Geometry check sheet. Reference: the model listing, model coordinates, mm. A direction names the side the tool comes from. Coordinates: 2 decimals unless noted, no trailing zeros. Order: outer loops, then holes, each group sorted by start corner. A loop starts at its lowest first (then second) coordinate and runs counter-clockwise, first axis right, second up. Notation, with made-up numbers: M -28.75,-32.75 L -2.75,-32.75 A27 cw -2.75,2.25 Z; hole C 18,7 d5. An arc over 180 degrees is marked long. One line per item, written item: value. Start each with the question number.
1) Sectioned sample at A-A, the plane z = -6.25. Enter the section's corners in (x, y), then the cut area to 3 significant figures.
2) Sectioned sample at C-C, the plane x = 1. Enter the section's corners in (y, z), then the cut area to 3 significant figures.
3) Go/stop test with flat-tipped pins: P1, Ø2.5, axis at x = 31.91, y = -16.6, coming from the +Z side; P2, Ø1.5, axis at x = 6.5, y = -8.5, coming from the -Z side; P3, Ø6, axis at x = -33, z = 1.5, coming from the +Y side; P4, Ø2, axis at y = 9, z = 1, coming from the -X side. Record where each tip stops, or that it passes through.
4) Draft check along X on faces 1 (the cylindrical face through (-21.994, -5.777, -6.627)), 2 (the flat face through (-5, 14, -5)), 3 (the cylindrical face through (-39.64, -14.05, 1.48)). Enter one of: pulls with the +X half, pulls with the -X half, needs draft (parallel to the pull), parting line crosses it, or undercut.
5) Sectioned sample at B-B, the plane z = 1.25. Enter the section's corners in (x, y).
6) Sectioned sample at D-D, the plane y = -16.6. Enter the section's corners in (x, z).
7) Access from +Z, -Z, +X, -X, +Y, -Y to the whole of each face (thin tool, end or side, straight path). Record for faces 4 (the cylindrical face through (-3.868, 15.826, -6.627)), 5 (the flat face through (-19.62, -8.49, -2.46)), 6 (the flat face through (-6.517, 16.457, -2.465)), 7 (the flat face through (-26.67, -2.66, -4.09)).
8) Thickness scan on L1, parallel to Z at x = -21.5, y = -4; L2, parallel to Z at x = -33.5, y = -10; L3, parallel to Y at x = -31.91, z = 2.1. Record the ranges inside material, lowest first. Write a range as from..to.
```python
from build123d import *

# Parameters (mm, degrees)
SKETCH1_R           = 2
SKETCH1_R_2         = 2.45
SKETCH1_R_3         = 4
BOSS_EXTRUDE1_DEPTH = 3
SKETCH2_R           = 1.05
BOSS_EXTRUDE2_DEPTH = 8.3
SKETCH2_3_R         = 1.05
CUT_EXTRUDE1_DEPTH  = 5


with BuildPart() as part:
    # Sketch1 → Boss-Extrude1 (new body)
    with BuildSketch(Plane.XY):
        with BuildLine():
            Line((-11.41, 37.5), (11.41, 37.5))
            ThreePointArc((11.41, 37.5), (17.8088531, 35.73800163), (22.403743203, 30.948748641))
            Line((22.403743203, 30.948748641), (39.989594287, -1.551251359))
            ThreePointArc((39.989594287, -1.551251359), (39.733852714, -13.8988531), (28.995851084, -20))
            Line((28.995851084, -20), (-28.995851084, -20))
            ThreePointArc((-28.995851084, -20), (-39.733852714, -13.8988531), (-39.989594287, -1.551251359))
            Line((-39.989594287, -1.551251359), (-22.403743203, 30.948748641))
            ThreePointArc((-22.403743203, 30.948748641), (-17.8088531, 35.73800163), (-11.41, 37.5))
        make_face()
        with Locations((-11.41, 25)):
            Circle(SKETCH1_R, mode=Mode.SUBTRACT)
        with Locations((11.41, 25)):
            Circle(SKETCH1_R, mode=Mode.SUBTRACT)
        with Locations((16.41, 0)):
            Circle(SKETCH1_R_2, mode=Mode.SUBTRACT)
        with Locations((0, 33.5)):
            Circle(SKETCH1_R, mode=Mode.SUBTRACT)
        with Locations((31.91, -16.6)):
            Circle(SKETCH1_R, mode=Mode.SUBTRACT)
        with Locations((-31.91, -16.6)):
            Circle(SKETCH1_R, mode=Mode.SUBTRACT)
        with Locations((-16.41, 0)):
            Circle(SKETCH1_R_3, mode=Mode.SUBTRACT)
    extrude(amount=BOSS_EXTRUDE1_DEPTH)

    # Sketch2 → Boss-Extrude2 (add)
    with BuildSketch(Plane(origin=(0, 0, 0), x_dir=(-1, 0, 0), z_dir=(0, 0, -1))):
        Polygon((0.324072443, 14.503290476), (3.47373173, 10.749672705), (8.069998389, 14.606398363), (4.920339102, 18.360016134), align=None)
        with Locations((4.004199133, 14.784657752)):
            Circle(SKETCH2_R, mode=Mode.SUBTRACT)
        Polygon((-2.088967553, 12.478509505), (1.060691735, 8.724891734), (3.47373173, 10.749672705), (0.324072443, 14.503290476), align=None)
        Polygon((4.920339102, 18.360016134), (8.069998389, 14.606398363), (10.483038385, 16.631179333), (7.333379097, 20.384797104), align=None)
        Polygon((18.06501047, -6.639536154), (15.651970474, -8.664317125), (18.801629762, -12.417934896), (21.214669758, -10.393153926), align=None)
        Polygon((22.661277129, -2.782810496), (18.06501047, -6.639536154), (21.214669758, -10.393153926), (25.810936416, -6.536428267), align=None)
        with Locations((22.130809726, -6.817795544)):
            Circle(SKETCH2_R, mode=Mode.SUBTRACT)
        Polygon((25.074317125, -0.758029526), (22.661277129, -2.782810496), (25.810936416, -6.536428267), (28.223976412, -4.511647297), align=None)
    extrude(amount=BOSS_EXTRUDE2_DEPTH)

    # Sketch2_3 → Cut-Extrude1 (cut)
    with BuildSketch(Plane(origin=(0, 0, 0), x_dir=(-1, 0, 0), z_dir=(0, 0, -1))):
        Polygon((0.324072443, 14.503290476), (3.47373173, 10.749672705), (8.069998389, 14.606398363), (4.920339102, 18.360016134), align=None)
        with Locations((4.004199133, 14.784657752)):
            Circle(SKETCH2_3_R, mode=Mode.SUBTRACT)
        Polygon((22.661277129, -2.782810496), (18.06501047, -6.639536154), (21.214669758, -10.393153926), (25.810936416, -6.536428267), align=None)
        with Locations((22.130809726, -6.817795544)):
            Circle(SKETCH2_3_R, mode=Mode.SUBTRACT)
    extrude(amount=CUT_EXTRUDE1_DEPTH, mode=Mode.SUBTRACT)


solid = part.part
```
Final values:
1. outline: M -28.22,-4.51 L -18.8,-12.42 L -15.65,-8.66 L -25.07,-0.76 Z; M -10.48,16.63 L -1.06,8.72 L 2.09,12.48 L -7.33,20.38 Z; hole C -22.13,-6.82 d2.1; hole C -4,14.78 d2.1
1. area: 114 mm^2
2. outline: M -20,0 L 11.18,0 L 11.18,-8.3 L 13.39,-8.3 L 13.39,0 L 31.77,0 L 31.77,3 L -20,3 Z; M 35.23,0 L 37.5,0 L 37.5,3 L 35.23,3 Z
2. area: 180 mm^2
3. P1: passes through
3. P2: stops at z = 0
3. P3: stops at y = 16.91
3. P4: stops at x = -34.82
4. face 1: undercut
4. face 2: needs draft
4. face 3: pulls with the -X half
5. outline: M -39.99,-1.55 A12.5 ccw -29,-20 L 29,-20 A12.5 ccw 39.99,-1.55 L 22.4,30.95 A12.5 ccw 11.41,37.5 L -11.41,37.5 A12.5 ccw -22.4,30.95 Z; hole C -31.91,-16.6 d4; hole C -16.41,0 d8; hole C -11.41,25 d4; hole C 0,33.5 d4; hole C 11.41,25 d4; hole C 16.41,0 d4.9; hole C 31.91,-16.6 d4
6. outline: M -37.57,0 L -33.91,0 L -33.91,3 L -37.57,3 Z; M -29.91,0 L 29.91,0 L 29.91,3 L -29.91,3 Z; M 33.91,0 L 37.57,0 L 37.57,3 L 33.91,3 Z
7. face 4: -Z
7. face 5: -X, +Y
7. face 6: +X, -Y
7. face 7: -Z, -X, +Y
8. L1: z = -8.3..-5, 0..3
8. L2: z = 0..3
8. L3: y = -19.66..-18.6, -14.6..13.38
